Part model, mm, in its own coordinate system. Face numbers are marked on the shaded views. A direction names the side the tool comes from. Coordinates: 2 decimals unless noted, no trailing zeros. Loops run counter-clockwise (first coordinate to the right, second up) from the corner with the lowest first, then second, coordinate; pieces in that order, holes last. Notation, with made-up numbers: (57, 32) - (68, 32) arc R17 ccw to (68, 36) - close; hole circle Ø4 at (75, -2.5). An arc over 180 degrees is marked (long way). Use a Markdown table: item, result. Add a question column.
1. Band-saw the part on A-A, the plane y = 146. Give the cut face in (x, z) (3 decimals), plus the area to 3 significant figures.
2. 3-axis set-ups, long thin cutter, end or side, ignore diameter. For the marked faces 1 and 2: which of +Z, -Z, +X, -X, +Y, -Y reach the whole face in a straight line?
3. Band-saw the part on B-B, the plane x = 73. Give the cut face in (y, z) (3 decimals).
4. Wall check: probe 1 along X at (y, z) = (52.5, -63.5) (3 decimals); probe 2 along Z at (x, y) = (65, 150) (3 decimals). Give the ranges that are in metal, low to high. Write a range as [from, to].
5. Drop a flat-ended pin along its axis: pin 1 (24 mm diameter, centred on y = 61, z = -74.5, fed in from +X) (3 decimals). Give the stop position or say it passes through.
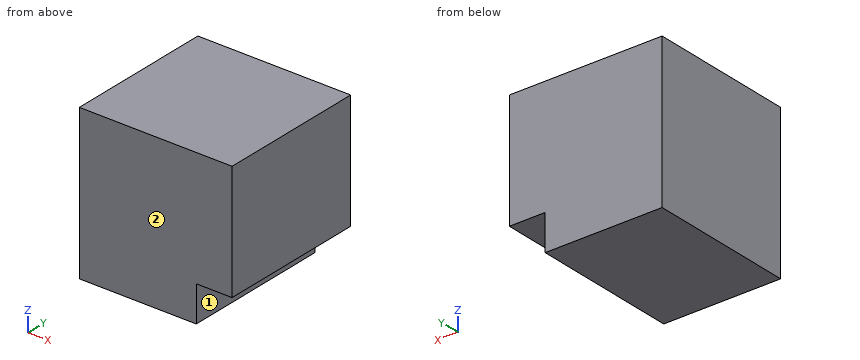
Autodesk Inventor part; units mm, degrees
ref_plane "YZ Plane" through (0, 0, 0) normal (1, 0, 0) x (0, 1, 0)
ref_plane "XZ Plane" through (0, 0, 0) normal (0, 1, 0) x (-1, 0, 0)
ref_plane "XY Plane" through (0, 0, 0) normal (0, 0, 1) x (1, 0, 0)
sketch "Sketch1" plane through (0, 0, 0) normal (0, 1, 0) x (-1, 0, 0)
  line L0 (101.6, -101.6) -> (-101.6, -101.6)
  line L1 (-101.6, -101.6) -> (-101.6, 101.6)
  line L2 (-101.6, 101.6) -> (101.6, 101.6)
  line L3 (101.6, 101.6) -> (101.6, -101.6)
  line L4 (101.6, -101.6) -> (-101.6, 101.6) construction
  line L5 (-101.6, -101.6) -> (101.6, 101.6) construction
  point P0 (0, 0)
  dimension "d0" = 203.2
  dimension "d1" = 203.2
extrude "Extrusion1" add sketch "Sketch1" along normal blind 196.85
sketch "Sketch2" plane through (0, 196.85, 0) normal (0, 1, 0) x (1, 0, 0)
  line L0 (101.6, -101.6) -> (101.6, 101.6)
  line L1 (101.6, 101.6) -> (53.975, 101.6)
  line L2 (53.975, 101.6) -> (53.975, 53.975)
  line L3 (53.975, 53.975) -> (101.6, 53.975)
  line L4 (101.6, 53.975) -> (101.6, 101.6)
  point P0 (0, 0)
  point P1 (101.6, 53.975)
  dimension "d4" = 47.625
  dimension "d5" = 47.625
extrude "Extrusion2" cut sketch "Sketch2" against normal up to surface (196.85 mm away)
properties part number "1-32" material "Limestone"
Geometry check:
| question | item | result |
|---|---|---|
| 1 | outline | (-101.6, -101.6) - (53.975, -101.6) - (53.975, -53.975) - (101.6, -53.975) - (101.6, 101.6) - (-101.6, 101.6) - close |
| 1 | area | 39,000 mm^2 |
| 2 | face 1 | -Z, +X, +Y, -Y |
| 2 | face 2 | +Z, -Z, +X, -X, -Y |
| 3 | outline | (0, -53.975) - (196.85, -53.975) - (196.85, 101.6) - (0, 101.6) - close |
| 4 | probe 1 | x = [-101.6, 53.975] |
| 4 | probe 2 | z = [-53.975, 101.6] |
| 5 | pin 1 | stops at x = 53.975 |
